Here's the drawing with two shaded views (mm, measured from the low corner). I have some questions. A direction names the side the tool comes from. Round coordinates to 2 decimals unless told otherwise and drop trailing zeros. Write each loop counter-clockwise with the first axis right and the second up, starting at its lowest first coordinate (ties: lowest second). Pieces come first, ordered by that corner, then holes. Notation, with made-up numbers: (4, 4.5) -> (62, 4.5) arc R20 ccw to (62, 28.5) -> close; hole circle Ø8 at (-35, 28.25). An arc over 180 degrees is marked (long way). Use CSV: the item, a comma, the result in double quotes.
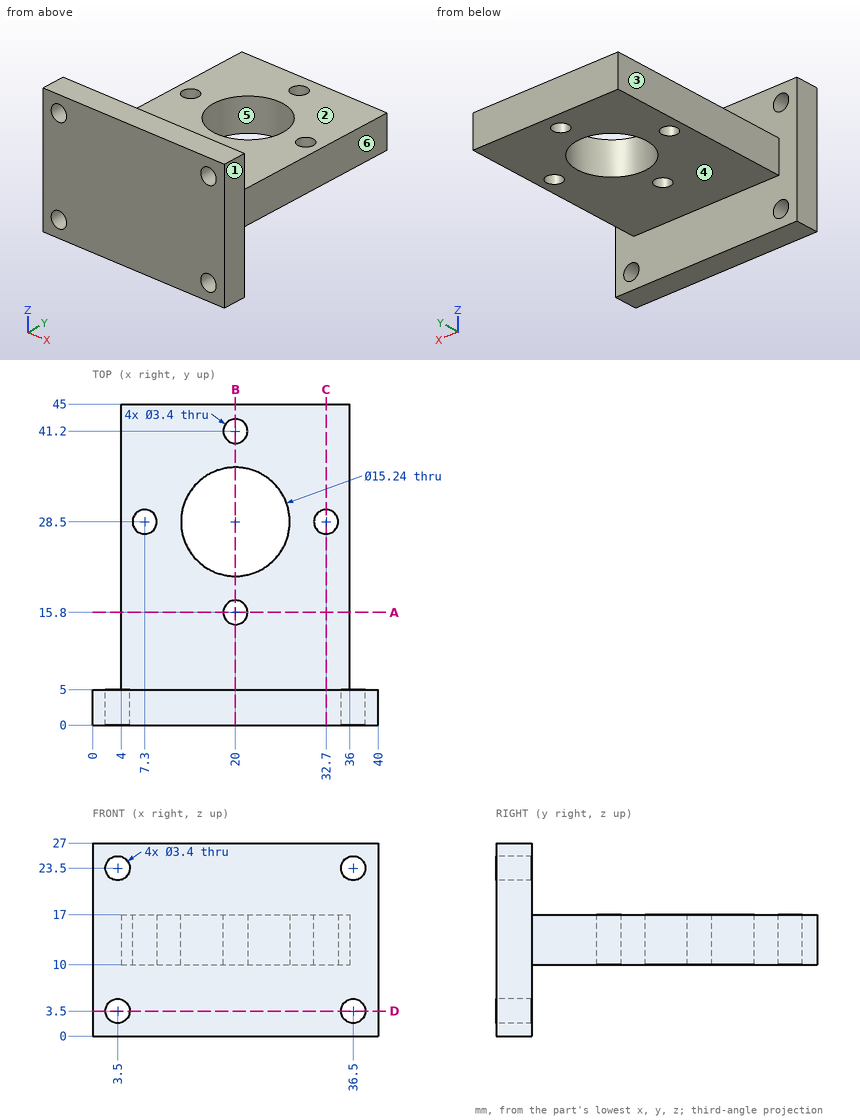
Q1. If we mould it in two halves opening along X, with no side actions, what happens to the marked faces 4, 5 and 6? For each: released by +X, released by -X, zero draft, split by the parting line, or undercut.
Resolved:
face 4,"zero draft"
face 5,"undercut"
face 6,"released by +X"
Q2. Please list where these lines run through material, in increasing order: probe 1 along X at (y, z) = (1.75, 3.5); probe 2 along Y at (x, z) = (20, 12); probe 3 along Y at (x, z) = (9.5, 7.5).
Resolved:
probe 1,"x = 0 to 1.8, 5.2 to 34.8, 38.2 to 40"
probe 2,"y = 0 to 14.1, 17.5 to 20.88, 36.12 to 39.5, 42.9 to 45"
probe 3,"y = 0 to 5"
Q3. Suppose I cut it at D-D (z = 3.5). Write out the boundary of the cut face in (x, y), and give its area (3 significant figures).
Resolved:
outline,"(0, 0) -> (1.8, 0) -> (1.8, 5) -> (0, 5) -> close; (5.2, 0) -> (34.8, 0) -> (34.8, 5) -> (5.2, 5) -> close; (38.2, 0) -> (40, 0) -> (40, 5) -> (38.2, 5) -> close"
area,"166 mm^2"
Q4. Suppose I cut it at B-B (x = 20). Write out the boundary of the cut face in (y, z), and give its area (3 significant figures).
Resolved:
outline,"(0, 0) -> (5, 0) -> (5, 10) -> (14.1, 10) -> (14.1, 17) -> (5, 17) -> (5, 27) -> (0, 27) -> close; (17.5, 10) -> (20.88, 10) -> (20.88, 17) -> (17.5, 17) -> close; (36.12, 10) -> (39.5, 10) -> (39.5, 17) -> (36.12, 17) -> close; (42.9, 10) -> (45, 10) -> (45, 17) -> (42.9, 17) -> close"
area,"261 mm^2"
Q5. Suppose I cut it at C-C (x = 32.7). Write out the boundary of the cut face in (y, z).
Resolved:
outline,"(0, 0) -> (5, 0) -> (5, 10) -> (26.8, 10) -> (26.8, 17) -> (5, 17) -> (5, 27) -> (0, 27) -> close; (30.2, 10) -> (45, 10) -> (45, 17) -> (30.2, 17) -> close"
Q6. Suppose I cut it at A-A (y = 15.8). Write out the boundary of the cut face in (x, z), and give its area (3 significant figures).
Resolved:
outline,"(4, 10) -> (18.3, 10) -> (18.3, 17) -> (4, 17) -> close; (21.7, 10) -> (36, 10) -> (36, 17) -> (21.7, 17) -> close"
area,"200 mm^2"
Q7. On a 3-axis mill with a long thin cutter (end or side, diameter ignored), from which of +Z, -Z, +X, -X, +Y, -Y can I reach the whole of each face in a straight line? I mean the marked faces 1, 2 and 3. Say none if no direction works.
Resolved:
face 1,"+Z, -Z, +X, +Y, -Y"
face 2,"+Z, +X, -X, +Y"
face 3,"+Z, -Z, -X, +Y"
Q8. Will these pins go through, and if not, where does the flat tip stop? P1, Ø1, axis at x = 23.5, z = 11.5, coming from the -Y side; P2, Ø5.5, axis at y = 22.5, z = 15, coming from the -X side; P3, Ø1, axis at y = 25, z = 15, coming from the +X side; P4, Ø9.5, axis at x = 21.5, y = 26, coming from the +Z side.
Resolved:
P1,"stops at y = 0"
P2,"stops at x = 4"
P3,"stops at x = 36"
P4,"stops at z = 17"
